from build123d import *

# Parameters (mm, degrees)
F0_W     = 10
F0_H     = 7
F1_DEPTH = 24
F2_DEPTH = 34


with BuildPart() as f1:
    # F0 (on Front) → F1 (new body)
    with BuildSketch(Plane.XZ):
        with BuildLine():
            ThreePointArc((-6.6169165431, 2.8701706491), (-11.6169165431, 5.485347467), (-16.6169165431, 2.8701706491))
            Line((-16.6169165431, 2.8701706491), (-6.6169165431, 2.8701706491))
        make_face()
        with BuildLine():
            Line((-6.6169165431, -4.1298293509), (-16.6169165431, -4.1298293509))
            ThreePointArc((-16.6169165431, -4.1298293509), (-11.6169165431, -6.1927828871), (-6.6169165431, -4.1298293509))
        make_face()
        with Locations((-11.6169165431, -0.6298293509)):
            Rectangle(F0_W, F0_H)
        with BuildLine():
            ThreePointArc((-12.7349732604, -1.6020070586), (-12.1521337532, 0.7992321504), (-10.1169165431, -0.6020324705))
            ThreePointArc((-10.1169165431, -0.6020324705), (-10.2156519221, -1.1372496806), (-10.4988598258, -1.6020070586))
            ThreePointArc((-10.4988598258, -1.6020070586), (-11.6169165431, -2.1020324705), (-12.7349732604, -1.6020070586))
        make_face(mode=Mode.SUBTRACT)
    extrude(amount=F1_DEPTH)

    # F0 (on Front) → F2 (join)
    with BuildSketch(Plane.XZ):
        with BuildLine():
            ThreePointArc((-10.4988598258, -1.6020070586), (-10.2156519221, -1.1372496806), (-10.1169165431, -0.6020324705))
            ThreePointArc((-10.1169165431, -0.6020324705), (-12.1521337532, 0.7992321504), (-12.7349732604, -1.6020070586))
            Line((-12.7349732604, -1.6020070586), (-11.6097875087, -1.6020070586))
            Line((-11.6097875087, -1.6020070586), (-10.4988598258, -1.6020070586))
        make_face()
    extrude(amount=F2_DEPTH)


solid = f1.part
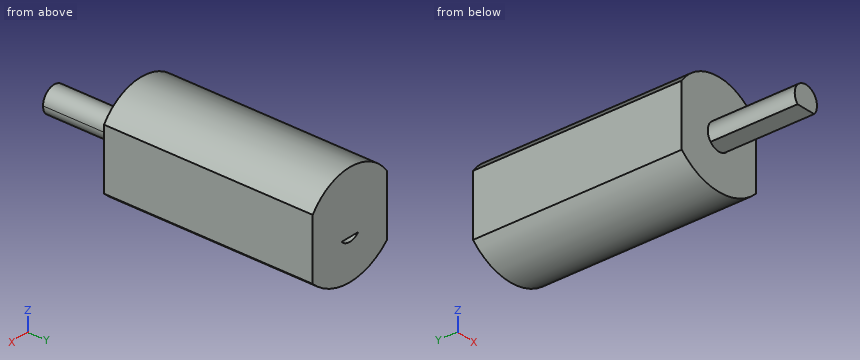
The listing builds one solid part. Answer for the finished solid, in the listing's coordinates (mm). Coordinates: 2 decimals unless noted, no trailing zeros. Loops run counter-clockwise (first coordinate to the right, second up) from the corner with the lowest first, then second, coordinate; pieces in that order, holes last. Notation, with made-up numbers: M -21.5,81 L 23.5,81 A33 ccw 23.5,111 Z; hole C 53.25,9.25 d6. An arc over 180 degrees is marked long. Answer in a Markdown table with one row per item.
1) Find section C-C (z = 2.5). Determine the outline of the cut face in (x, y).
Answers below:
| item | result |
|---|---|
| outline | M -16.62,-24 L -6.62,-24 L -6.62,0 L -16.62,0 Z |
2) Find section B-B (x = -12). Determine the outline of the cut face in (y, z), then the cut area to 3 significant figures.
Answers below:
| item | result |
|---|---|
| outline | M -34,-1.6 L 0,-1.6 L 0,5.47 L -24,5.47 L -24,0.85 L -34,0.85 Z; M -24,-6.18 L 0,-6.18 L 0,-2.05 L -24,-2.05 Z |
| area | 293 mm^2 |
3) Find section A-A (y = -14). Determine the outline of the cut face in (x, z).
Answers below:
| item | result |
|---|---|
| outline | M -16.62,-4.13 A7.09 ccw -6.62,-4.13 L -6.62,2.87 A6.09 ccw -16.62,2.87 Z; hole M -12.73,-1.6 A1.5 ccw -10.5,-1.6 Z |
4) Find the intervals of material crossed by probe 1 along Y at (x, z) = (-12.25, 4.5); probe 2 along Z at (x, y) = (-11.5, -7.5); probe 3 along Z at (x, y) = (-12.25, -16), in increasing order.
Answers below:
| item | result |
|---|---|
| probe 1 | -24 to 0 |
| probe 2 | -6.19 to -2.1, -1.6 to 5.48 |
| probe 3 | -6.16 to -1.96, -1.6 to 5.45 |
5) Given pin 1 (0.7 mm diameter, centred on x = -11, y = -25.5, fed in from -Z), flat-ended and moving along its own axis, determine where the tip first touches the part or whether it passes through.
Answers below:
| item | result |
|---|---|
| pin 1 | z = -1.6 |
6) Find section D-D (y = -28). Determine the outline of the cut face in (x, z), then the cut area to 3 significant figures.
Answers below:
| item | result |
|---|---|
| outline | M -12.73,-1.6 L -10.5,-1.6 A1.5 ccw long Z |
| area | 6.29 mm^2 |
